Build history of the part. All positions in model axes, mm. A direction names the side the tool comes from. Give positions to 0.01 mm unless a question says otherwise; leave off trailing zeros. Write each loop counter-clockwise with the first axis right and the second up, starting at its lowest first coordinate (ties: lowest second). Pieces come first, ordered by that corner, then holes. Notation, with made-up numbers: (80, -11.5) -> (123, -11.5) arc R29 cw to (123, 20.5) -> close; hole circle Ø4 at (-39, 42.25). An arc over 180 degrees is marked (long way). Put each result on its own line as item: value.
from build123d import *

# Parameters (mm, degrees)
SKETCH_1_R          = 5.25
EXTRUDE_1_DEPTH     = 10
SKETCH_2_R          = 5
CUT_EXTRUDE_1_DEPTH = 10
CUT_EXTRUDE_2_DEPTH = 10


with BuildPart() as part:
    # 草图1 → 凸台-拉伸1 (new body)
    with BuildSketch(Plane.XY):
        with BuildLine():
            Line((-100, 10), (100, 10))
            Line((100, 10), (125, 10))
            ThreePointArc((125, 10), (135, 0), (125, -10))
            Line((125, -10), (100, -10))
            Line((100, -10), (-100, -10))
            ThreePointArc((-100, -10), (-110, 0), (-100, 10))
        make_face()
        with Locations((-100, 0)):
            Circle(SKETCH_1_R, mode=Mode.SUBTRACT)
        with Locations((100, 0)):
            Circle(SKETCH_1_R, mode=Mode.SUBTRACT)
    extrude(amount=EXTRUDE_1_DEPTH)

    # 草图2 → 切除-拉伸1 (cut)
    with BuildSketch(Plane.XY.offset(10)):
        Circle(SKETCH_2_R)
    extrude(amount=-CUT_EXTRUDE_1_DEPTH, mode=Mode.SUBTRACT)

    # 草图4 → 切除-拉伸2 (cut)
    with BuildSketch(Plane.XY.offset(10)):
        with BuildLine():
            Line((-80, 5), (-20, 5))
            ThreePointArc((-20, 5), (-15, 0), (-20, -5))
            Line((-20, -5), (-80, -5))
            ThreePointArc((-80, -5), (-85, 0), (-80, 5))
        make_face()
        with BuildLine():
            Line((20, 5), (80, 5))
            ThreePointArc((80, 5), (85, 0), (80, -5))
            Line((80, -5), (20, -5))
            ThreePointArc((20, -5), (15, 0), (20, 5))
        make_face()
    extrude(amount=-CUT_EXTRUDE_2_DEPTH, mode=Mode.SUBTRACT)


solid = part.part
1) Tool access for faces 4 (the flat face through (11, 10, 5)), 5 (the cylindrical face through (-15, 0, 5)): list every direction of +Z, -Z, +X, -X, +Y, -Y with a clear straight run to the whole face (end or side of a thin tool).
Filled sheet:
face 4: +Z, -Z, +X, -X, +Y
face 5: +Z, -Z
2) Slice it at D-D (x = -69.5). Write the cut outline in (y, z).
Filled sheet:
outline: (-10, 0) -> (-5, 0) -> (-5, 10) -> (-10, 10) -> close; (5, 0) -> (10, 0) -> (10, 10) -> (5, 10) -> close
3) Slice it at B-B (z = 5.5). Write the cut outline in (x, y), plus the area to 3 significant figures.
Filled sheet:
outline: (-100, -10) -> (125, -10) arc R10 ccw to (125, 10) -> (-100, 10) arc R10 ccw to start; hole circle Ø10.5 at (-100, 0); hole (-80, -5) -> (-20, -5) arc R5 ccw to (-20, 5) -> (-80, 5) arc R5 ccw to start; hole circle Ø10 at (0, 0); hole (20, -5) -> (80, -5) arc R5 ccw to (80, 5) -> (20, 5) arc R5 ccw to start; hole circle Ø10.5 at (100, 0)
area: 3,210 mm2
4) Pin check, flat tips, straight feed: pin 1 (2 mm diameter, centred on y = -3.5, z = 2, fed in from -X); pin 2 (8.5 mm diameter, centred on x = -100, y = 0, fed in from +Z). Stop position of each tip, or through.
Filled sheet:
pin 1: x = -109.68
pin 2: through
5) Slice it at C-C (y = 3). Write the cut outline in (x, z), plus the area to 3 significant figures.
Filled sheet:
outline: (-109.54, 0) -> (-104.31, 0) -> (-104.31, 10) -> (-109.54, 10) -> close; (-95.69, 0) -> (-84, 0) -> (-84, 10) -> (-95.69, 10) -> close; (-16, 0) -> (-4, 0) -> (-4, 10) -> (-16, 10) -> close; (4, 0) -> (16, 0) -> (16, 10) -> (4, 10) -> close; (84, 0) -> (95.69, 0) -> (95.69, 10) -> (84, 10) -> close; (104.31, 0) -> (134.54, 0) -> (134.54, 10) -> (104.31, 10) -> close
area: 828 mm2
6) Pull direction X, two halves, no side cores. Call faces 1 (the cylindrical face through (135, 0, 5)), 2 (the flat face through (14, 0, 10)), 3 (the flat face through (50, -5, 5)): released by +X, released by -X, zero draft, split by the parting line, or undercut.
Filled sheet:
face 1: released by +X
face 2: zero draft
face 3: undercut
7) Slice it at A-A (x = 100). Write the cut outline in (y, z), plus the area to 3 significant figures.
Filled sheet:
outline: (-10, 0) -> (-5.25, 0) -> (-5.25, 10) -> (-10, 10) -> close; (5.25, 0) -> (10, 0) -> (10, 10) -> (5.25, 10) -> close
area: 95.0 mm2
8) Wall check: L1, parallel to Y at x = -100, z = 6; L2, parallel to Y at x = 43.5, z = 1.5; L3, parallel to X at y = 1.5, z = 4.5. Give the ranges that are in metal, low to high.
Filled sheet:
L1: -10 to -5.25, 5.25 to 10
L2: -10 to -5, 5 to 10
L3: -109.89 to -105.03, -94.97 to -84.77, -15.23 to -4.77, 4.77 to 15.23, 84.77 to 94.97, 105.03 to 134.89
